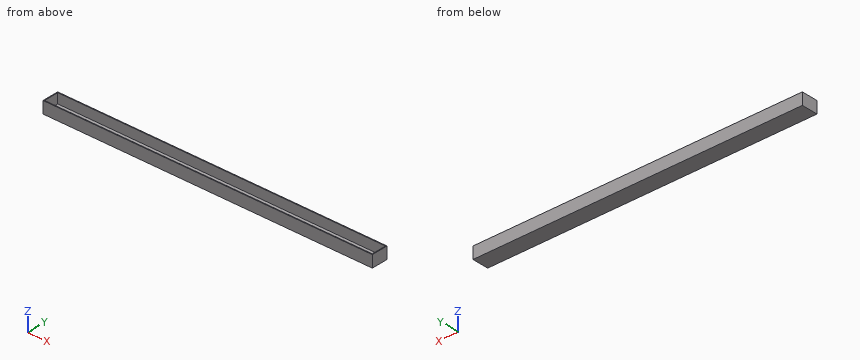
```python
from build123d import *

# Parameters (mm, degrees)
F0_W     = 100
F0_H     = 5
F1_DEPTH = 0.6
F2_W     = 100
F2_H     = 5
F4_DEPTH = 3
F3_W     = 99.5
F3_H     = 4.5
F5_DEPTH = 25


with BuildPart() as f1:
    # F0 (on Top) → F1 (new body)
    with BuildSketch(Plane.XY):
        Rectangle(F0_W, F0_H)
    extrude(amount=F1_DEPTH)

    # F2 (on face) → F4 (join)
    with BuildSketch(Plane.XY.offset(0.6)):
        Rectangle(F2_W, F2_H)
    extrude(amount=F4_DEPTH)

    # F3 (on face) → F5 (cut)
    with BuildSketch(Plane.XY.offset(0.6)):
        Rectangle(F3_W, F3_H)
    extrude(amount=F5_DEPTH, mode=Mode.SUBTRACT)


solid = f1.part
```
Model file for the job. Use its own axes, mm. Coordinates: 2 decimals unless noted, no trailing zeros. Order: outer loops, then holes, each group sorted by start corner. A loop starts at its lowest first (then second) coordinate and runs counter-clockwise, first axis right, second up. Notation, with made-up numbers: (57, -27) -> (89, -27) arc R17 cw to (89, 4) -> close; hole circle Ø11 at (-27.75, 17). An arc over 180 degrees is marked (long way). Return JSON: item names as keys, results as strings.
Item 1: Slice it at B-B (y = 0.7). Write the cut outline in (x, z), then the cut area to 3 significant figures.
Model answer:
{"outline": "(-50, 0) -> (50, 0) -> (50, 3.6) -> (49.75, 3.6) -> (49.75, 0.6) -> (-49.75, 0.6) -> (-49.75, 3.6) -> (-50, 3.6) -> close", "area": "61.5 mm²"}
Item 2: Slice it at C-C (x = -5.5). Write the cut outline in (y, z), then the cut area to 3 significant figures.
Model answer:
{"outline": "(-2.5, 0) -> (2.5, 0) -> (2.5, 3.6) -> (2.25, 3.6) -> (2.25, 0.6) -> (-2.25, 0.6) -> (-2.25, 3.6) -> (-2.5, 3.6) -> close", "area": "4.50 mm²"}
Item 3: Slice it at A-A (z = 2.75). Write the cut outline in (x, y).
Model answer:
{"outline": "(-50, -2.5) -> (50, -2.5) -> (50, 2.5) -> (-50, 2.5) -> close; hole (-49.75, -2.25) -> (49.75, -2.25) -> (49.75, 2.25) -> (-49.75, 2.25) -> close"}
Item 4: Pin check, flat tip, straight feed: P1, Ø2, axis at x = -1.5, y = -0.5, coming from the +Z side. Stop position of the tip, or through.
Model answer:
{"P1": "stops at z = 0.6"}
Item 5: Wall check: line 1 along Y through (x, z) = (-31, 2.1); line 2 along X through (y, z) = (-1.75, 2.8); line 3 along Z through (x, y) = (27, -0.6). Give the ranges that are in metal, low to high. Write a range as from..to.
Model answer:
{"line 1": "y = -2.5..-2.25, 2.25..2.5", "line 2": "x = -50..-49.75, 49.75..50", "line 3": "z = 0..0.6"}
